from build123d import *

# Parameters (mm, degrees)
EXTRUDE_1_DEPTH     = 15
SKETCH_2_R          = 2.7
CUT_EXTRUDE_1_DEPTH = 3.5
SKETCH_3_R          = 1.65
CUT_EXTRUDE_2_DEPTH = 25.924887161
FILLET_1_R          = 2
CHAMFER_1_SIZE      = 0.5


# Read off the part's stored shape, not the designer's step: 填料-伸長1
with BuildPart() as part:
    # 填料-伸長1 outline → 填料-伸長1 (new body)
    with BuildSketch(Plane.XY):
        Polygon((0, 0), (0, 12), (-18, 12), (-18, 0), (-15, 0), (-15, 8), (-3, 8), (-3, 0), align=None)
    extrude(amount=EXTRUDE_1_DEPTH)

    # 草圖2 → 除料-伸長1 (cut)
    with BuildSketch(Plane(origin=(0, 12, 0), x_dir=(1, 0, 0), z_dir=(0, 1, 0))):
        with Locations(Location((-9, -7.5, 0), (0, 0, 180))):
            Circle(SKETCH_2_R)
    extrude(amount=-CUT_EXTRUDE_1_DEPTH, mode=Mode.SUBTRACT)

    # 草圖3 → 除料-伸長2 (cut, through all)
    with BuildSketch(Plane(origin=(0, 8.5, 0), x_dir=(1, 0, 0), z_dir=(0, 1, 0))):
        with Locations(Location((-9, -7.5, 0), (0, 0, 180))):
            Circle(SKETCH_3_R)
    extrude(amount=-CUT_EXTRUDE_2_DEPTH, mode=Mode.SUBTRACT)

    # 圓角1
    fillet_1_edges = [part.edges().sort_by_distance(p)[0] for p in [
        (-18, 12, 7.5),
        (0, 12, 7.5),
    ]]
    fillet(fillet_1_edges, radius=FILLET_1_R)

    # 導角1
    chamfer_1_edges = [part.edges().sort_by_distance(p)[0] for p in [
        (-6.3, 12, 7.5),
    ]]
    chamfer(chamfer_1_edges, length=CHAMFER_1_SIZE)


solid = part.part
Work out the finished part from the listing and answer in its coordinate system (mm). A direction names the side the tool comes from. Give positions to 0.01 mm unless a question says otherwise; leave off trailing zeros. Loops run counter-clockwise (first coordinate to the right, second up) from the corner with the lowest first, then second, coordinate; pieces in that order, holes last. Notation, with made-up numbers: (21.5, 77.5) -> (34.5, 77.5) arc R20 ccw to (34.5, 108.5) -> close; hole circle Ø7 at (-30, 23.25). An arc over 180 degrees is marked (long way). Use a Markdown table: item, result. Add a question column.
1. Section D-D on z = 11.5 is taken. Determine the outline of the cut face in (x, y), and give its area (3 significant figures).
2. Section B-B on z = 7.5 is taken. Determine the outline of the cut face in (x, y).
3. For faces 4 (the flat face through (-9.1, 8, 5.7)), 5 (the cylindrical face through (-17.4, 11.43, 7.6)), 6 (the cylindrical face through (-10.246, 10.021, 5.105)), determine the directions among +Z, -Z, +X, -X, +Y, -Y from which every point of the face is accessible in a straight line to the end or side of a thin tool.
4. Determine the mould class of faces 1 (the flat face through (-3, 4, 7)), 2 (the flat face through (0, 5, 7)), 3 (the flat face through (-9, 9, 0)) for opening direction X: released by +X, released by -X, zero draft, split by the parting line, or undercut.
5. Section A-A on x = -9 is taken. Determine the outline of the cut face in (y, z), and give its area (3 significant figures).
6. Find the intervals of material crossed by probe 1 along X at (y, z) = (7.25, 4.25); probe 2 along Z at (x, y) = (-9, 8.3); probe 3 along Y at (x, z) = (-11.5, 12), in increasing order.
7. A flat-ended cylindrical pin translates along its axis: pin 1 Ø3.5 at (x, z) = (-9.5, 9) entering from -Y. Find the tip coordinate at first contact, or state that the pin passes through.
8. Section C-C on y = 9 is taken. Determine the outline of the cut face in (x, z).
Results below:
| question | item | result |
|---|---|---|
| 1 | outline | (-18, 0) -> (-15, 0) -> (-15, 8) -> (-3, 8) -> (-3, 0) -> (0, 0) -> (0, 10) arc R2 ccw to (-2, 12) -> (-16, 12) arc R2 ccw to (-18, 10) -> close |
| 1 | area | 118 mm^2 |
| 2 | outline | (-18, 0) -> (-15, 0) -> (-15, 8) -> (-10.65, 8) -> (-10.65, 8.5) -> (-11.7, 8.5) -> (-11.7, 11.5) -> (-12.2, 12) -> (-16, 12) arc R2 ccw to (-18, 10) -> close; (-7.35, 8) -> (-3, 8) -> (-3, 0) -> (0, 0) -> (0, 10) arc R2 ccw to (-2, 12) -> (-5.8, 12) -> (-6.3, 11.5) -> (-6.3, 8.5) -> (-7.35, 8.5) -> close |
| 3 | face 4 | +Z, -Z, -Y |
| 3 | face 5 | +Z, -Z, -X, +Y |
| 3 | face 6 | +Y |
| 4 | face 1 | undercut |
| 4 | face 2 | released by +X |
| 4 | face 3 | zero draft |
| 5 | outline | (8, 0) -> (12, 0) -> (12, 4.3) -> (11.5, 4.8) -> (8.5, 4.8) -> (8.5, 5.85) -> (8, 5.85) -> close; (8, 9.15) -> (8.5, 9.15) -> (8.5, 10.2) -> (11.5, 10.2) -> (12, 10.7) -> (12, 15) -> (8, 15) -> close |
| 5 | area | 39.2 mm^2 |
| 6 | probe 1 | x = -18 to -15, -3 to 0 |
| 6 | probe 2 | z = 0 to 5.85, 9.15 to 15 |
| 6 | probe 3 | y = 8 to 12 |
| 7 | pin 1 | stops at y = 8 |
| 8 | outline | (-18, 0) -> (0, 0) -> (0, 15) -> (-18, 15) -> close; hole circle Ø5.4 at (-9, 7.5) |
